from build123d import *
from OCP.BRepFilletAPI import BRepFilletAPI_MakeChamfer

# Parameters (mm, degrees)
SKETCH_1_R          = 10
EXTRUDE_1_DEPTH     = 20
SKETCH_7_R          = 1.55
CUT_EXTRUDE_2_DEPTH = 35.369317712
SKETCH_9_W          = 3
SKETCH_9_H          = 40
EXTRUDE_2_DEPTH     = 15
SKETCH_10_R         = 1.55
CUT_EXTRUDE_3_DEPTH = 49.440685517
CHAMFER_1_SIZE      = 5
CHAMFER_1_SIZE2     = 8.660254038
FILLET_1_R          = 5


with BuildPart() as part:
    # 草图1 → 凸台-拉伸1 (new, symmetric)
    with BuildSketch(Plane(origin=(0, 0, 0), x_dir=(1, 0, 0), z_dir=(0, 1, 0))):
        with BuildLine():
            Line((-12.5, -25), (12.5, -25))
            Line((12.5, -25), (12.5, 0))
            ThreePointArc((12.5, 0), (0, 12.5), (-12.5, 0))
            Line((-12.5, 0), (-12.5, -25))
        make_face()
        with Locations(Location((0, 0, 0), (0, 0, 270))):
            Circle(SKETCH_1_R, mode=Mode.SUBTRACT)
    extrude(amount=EXTRUDE_1_DEPTH, both=True)

    # 草图7 → 切除-拉伸2 (cut, through all)
    with BuildSketch(Plane.XY):
        with Locations(Location((0, -12, 0), (0, 0, 90))):
            Circle(SKETCH_7_R)
        with Locations(Location((0, 12, 0), (0, 0, 90))):
            Circle(SKETCH_7_R)
    extrude(amount=-CUT_EXTRUDE_2_DEPTH, mode=Mode.SUBTRACT)

    # 草图9 → 凸台-拉伸2 (add)
    with BuildSketch(Plane(origin=(12.5, 0, 0), x_dir=(0, 0, -1), z_dir=(1, 0, 0))):
        with Locations((-23.5, 0)):
            Rectangle(SKETCH_9_W, SKETCH_9_H)
    extrude_2 = extrude(amount=EXTRUDE_2_DEPTH)

    # 草图10 → 切除-拉伸3 (cut, through all)
    with BuildSketch(Plane(origin=(0, 0, 22), x_dir=(-1, 0, 0), z_dir=(0, 0, -1))):
        with Locations((-23.5, 15)):
            Circle(SKETCH_10_R)
        with Locations(Location((-23.5, -15, 0), (0, 0, 180))):
            Circle(SKETCH_10_R)
    cut_extrude_3 = extrude(amount=-CUT_EXTRUDE_3_DEPTH, mode=Mode.SUBTRACT)

    # 镜向6: 凸台-拉伸2, 切除-拉伸3 across plane
    add(extrude_2.mirror(Plane(origin=(0, 0, 0), x_dir=(0, 0, 1), z_dir=(1, 0, 0))))
    add(cut_extrude_3.mirror(Plane(origin=(0, 0, 0), x_dir=(0, 0, 1), z_dir=(1, 0, 0))), mode=Mode.SUBTRACT)

    # 倒角1: one chamfer whose edges measure the first distance from different faces: ONE call of the kernel's chamfer builder (chamfer() names one face for all edges)
    chamfer_1_edges_1 = [part.edges().sort_by_distance(p)[0] for p in [
        (12.5, 0, 22),
    ]]
    chamfer_1_side_1 = [part.faces().sort_by_distance(p)[0] for p in [
        (19.909671201, 0, 22),
    ]]
    chamfer_1_edges_2 = [part.edges().sort_by_distance(p)[0] for p in [
        (-12.5, 0, 22),
    ]]
    chamfer_1_side_2 = [part.faces().sort_by_distance(p)[0] for p in [
        (-19.909671201, 0, 22),
    ]]
    chamfer_1 = BRepFilletAPI_MakeChamfer(part.part.solid().wrapped)
    for e in chamfer_1_edges_1:
        chamfer_1.Add(CHAMFER_1_SIZE, CHAMFER_1_SIZE2, e.wrapped, chamfer_1_side_1[0].wrapped)  # the first distance lies on this face
    for e in chamfer_1_edges_2:
        chamfer_1.Add(CHAMFER_1_SIZE, CHAMFER_1_SIZE2, e.wrapped, chamfer_1_side_2[0].wrapped)  # the first distance lies on this face
    add(Compound.cast(chamfer_1.Shape()), mode=Mode.REPLACE)

    # 圆角1
    fillet_1_edges = [part.edges().sort_by_distance(p)[0] for p in [
        (27.5, -20, 23.5),
        (27.5, 20, 23.5),
        (-27.5, 20, 23.5),
        (-27.5, -20, 23.5),
    ]]
    fillet(fillet_1_edges, radius=FILLET_1_R)


solid = part.part
For this review, take the finished solid that the model builds, in its own axes (mm). A direction names the side the tool comes from. Coordinates: 2 decimals unless noted, no trailing zeros. Loops run counter-clockwise (first coordinate to the right, second up) from the corner with the lowest first, then second, coordinate; pieces in that order, holes last. Notation, with made-up numbers: (39, 0) - (69, 0) arc R9 ccw to (69, 4) - close; hole circle Ø10 at (-9, -20.75). An arc over 180 degrees is marked (long way). Return JSON: item names as keys, results as strings.
Item 1: Take a section at C-C (x = 9). Give the boundary of the cut face in (y, z).
Determined:
{"outline": "(-20, -8.67) - (20, -8.67) - (20, -4.36) - (-20, -4.36) - close; (-20, 4.36) - (20, 4.36) - (20, 25) - (-20, 25) - close"}
Item 2: Take a section at B-B (x = 0). Give the boundary of the cut face in (y, z), then the cut area to 4 significant figures.
Determined:
{"outline": "(-20, -12.5) - (-13.55, -12.5) - (-13.55, -10) - (-20, -10) - close; (-20, 10) - (20, 10) - (20, 25) - (-20, 25) - close; (-10.45, -12.5) - (10.45, -12.5) - (10.45, -10) - (-10.45, -10) - close; (13.55, -12.5) - (20, -12.5) - (20, -10) - (13.55, -10) - close", "area": "684.5 mm2"}
Item 3: Mouldability with a two-part tool opening along X and no side actions: class faces 4 (the cylindrical face through (-0.07, -13.55, -11.17)), 5 (the flat face through (12.5, 0, 7)), 6 (the flat face through (-27.5, 0, 24)) as pulls with the +X half, pulls with the -X half, needs draft (parallel to the pull), parting line crosses it, or undercut.
Determined:
{"face 4": "undercut", "face 5": "pulls with the +X half", "face 6": "pulls with the -X half"}
Item 4: For faces 1 (the cylindrical face through (3, -0.28, 9.54)), 2 (the flat face through (22, 0, 22)), 3 (the flat face through (-12.5, 0, 7)), list the 3-axis set-ups (+Z, -Z, +X, -X, +Y, -Y) from which the entire face can be reached by the end or side of a thin tool; tool diameter is ignored.
Determined:
{"face 1": "+Y, -Y", "face 2": "-Z, +X, +Y, -Y", "face 3": "-Z, -X, +Y, -Y"}
Item 5: For line 1 (X direction, y = -15, z = 23.9); line 2 (X direction, y = 11, z = 0); line 3 (Z direction, x = 0, y = -5.5), list the stretches that pass through material, from the lowest coordinate up.
Determined:
{"line 1": "x = -27.5 to -25.05, -21.95 to 21.95, 25.05 to 27.5", "line 2": "x = -12.5 to -10, 10 to 12.5", "line 3": "z = -12.5 to -10, 10 to 25"}
Item 6: Take a section at D-D (x = -23.5). Give the boundary of the cut face in (y, z).
Determined:
{"outline": "(-19.9, 22) - (-16.55, 22) - (-16.55, 25) - (-19.9, 25) - close; (-13.45, 22) - (13.45, 22) - (13.45, 25) - (-13.45, 25) - close; (16.55, 22) - (19.9, 22) - (19.9, 25) - (16.55, 25) - close"}
Item 7: Take a section at A-A (y = -8). Give the boundary of the cut face in (x, z), then the cut area to 3 significant figures.
Determined:
{"outline": "(-27.5, 22) - (-17.5, 22) - (-12.5, 13.34) - (-12.5, 0) arc R12.5 ccw to (12.5, 0) - (12.5, 13.34) - (17.5, 22) - (27.5, 22) - (27.5, 25) - (-27.5, 25) - close; hole circle Ø20 at (0, 0)", "area": "690 mm2"}
Item 8: Insertion check: pin 1 (3 mm diameter, centred on x = -25, y = -4, fed in from -Z); pin 2 (8 mm diameter, centred on y = 2, z = -5.5, fed in from -X); pin 3 (12 mm diameter, centred on y = -3.5, z = -1.5, fed in from +X); pin 4 (18 mm diameter, centred on x = 0, z = 0, fed in from -Y). Each pin has a flat end and moves straight along its axis. Give the tip position at first contact, or say it passes through.
Determined:
{"pin 1": "stops at z = 22", "pin 2": "stops at x = -12.41", "pin 3": "stops at x = 12.5", "pin 4": "passes through"}
